Can you work these out from the model? Positions are in its coordinate system, mm. Face numbers are marked on the shaded views. Give positions to 0.01 mm unless a question says otherwise; leave off trailing zeros. Order: outer loops, then holes, each group sorted by start corner. A loop starts at its lowest first (then second) coordinate and runs counter-clockwise, first axis right, second up. Notation, with made-up numbers: (-23, 49) - (12, 49) arc R7 ccw to (12, 60) - close; hole circle Ø7 at (78, 1.25). An arc over 180 degrees is marked (long way). Use one line per item in the form item = value. Start each with the question number.
1) We'd pull the mould along X, two halves only. Please class the marked faces 1, 2, 3 and 4: released by +X, released by -X, zero draft, split by the parting line, or undercut.
2) For pin 1 (6.5 mm diameter, centred on x = -71, z = 9.25, fed in from -Y); pin 2 (1.5 mm diameter, centred on x = -41.5, z = -9.5, fed in from +Y); pin 3 (4.5 mm diameter, centred on x = 71, z = -50.75, fed in from +Y), each with a flat end and sliding along its axis, tell me the tip position at first contact or that it passes through.
3) Suppose I cut it at A-A, the plane x = -71. Write out the boundary of the cut face in (y, z).
4) Suppose I cut it at B-B, the plane y = 3. Write out the boundary of the cut face in (x, z), and give its area (3 significant figures).
5) Please list where these lines run through material, in increasing order: probe 1 along Z at (x, y) = (71, 6); probe 2 along Z at (x, y) = (61.5, 8.25); probe 3 along Z at (x, y) = (-42.5, 4.5).
6) Suppose I cut it at D-D, the plane x = 65. Write out the boundary of the cut face in (y, z).
7) Suppose I cut it at C-C, the plane z = -50.75. Write out the boundary of the cut face in (x, y).
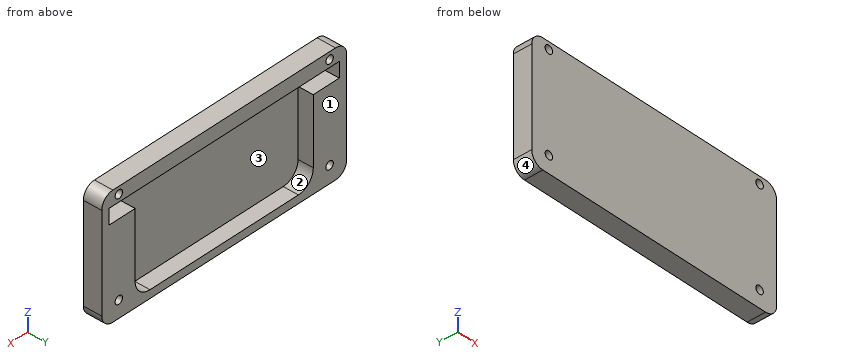
```python
from build123d import *

# Parameters (mm, degrees)
SKETCH_1_W      = 165
SKETCH_1_H      = 75
SKETCH_1_R      = 2.5
EXTRUDE_1_DEPTH = 9.5
EXTRUDE_START   = -2
SKETCH_1_2_W    = 165
SKETCH_1_2_H    = 75
SKETCH_1_2_R    = 2.5
EXTRUDE_2_DEPTH = 2
FILLET_1_R      = 10
FILLET_2_R      = 7.5


with BuildPart() as part:
    # Sketch 1 → Extrude 1 (new body)
    with BuildSketch(Plane(origin=(0, 0, 0), x_dir=(1, 0, 0), z_dir=(0, 1, 0))):
        with Locations((0, 23.75)):
            Rectangle(SKETCH_1_W, SKETCH_1_H)
        with Locations(Location((-71, -9.25, 0), (0, 0, 270))):
            Circle(SKETCH_1_R, mode=Mode.SUBTRACT)
        with Locations(Location((-71, 50.75, 0), (0, 0, 270))):
            Circle(SKETCH_1_R, mode=Mode.SUBTRACT)
        with Locations(Location((71, -9.25, 0), (0, 0, 90))):
            Circle(SKETCH_1_R, mode=Mode.SUBTRACT)
        with Locations(Location((71, 50.75, 0), (0, 0, 90))):
            Circle(SKETCH_1_R, mode=Mode.SUBTRACT)
        Polygon((77.5, -4.75), (-77.5, -4.75), (-77.5, 4.75), (-60, 4.75), (-60, 56.25), (60, 56.25), (60, 4.75), (77.5, 4.75), align=None, mode=Mode.SUBTRACT)
    extrude(amount=EXTRUDE_1_DEPTH)

    # Sketch 1_2 → Extrude 2 (add)
    # profile 1 of 2: a face of its own
    with BuildSketch(Plane(origin=(0, 0, 0), x_dir=(1, 0, 0), z_dir=(0, 1, 0)).offset(EXTRUDE_START)):
        with Locations((0, 23.75)):
            Rectangle(SKETCH_1_2_W, SKETCH_1_2_H)
        with Locations(Location((71, -9.25, 0), (0, 0, 90))):
            Circle(SKETCH_1_2_R, mode=Mode.SUBTRACT)
        with Locations(Location((-71, 50.75, 0), (0, 0, 270))):
            Circle(SKETCH_1_2_R, mode=Mode.SUBTRACT)
        with Locations(Location((-71, -9.25, 0), (0, 0, 270))):
            Circle(SKETCH_1_2_R, mode=Mode.SUBTRACT)
        with Locations(Location((71, 50.75, 0), (0, 0, 90))):
            Circle(SKETCH_1_2_R, mode=Mode.SUBTRACT)
        Polygon((77.5, -4.75), (77.5, 4.75), (60, 4.75), (60, 56.25), (-60, 56.25), (-60, 4.75), (-77.5, 4.75), (-77.5, -4.75), align=None, mode=Mode.SUBTRACT)
    # profile 2 of 2: a face of its own
    with BuildSketch(Plane(origin=(0, 0, 0), x_dir=(1, 0, 0), z_dir=(0, 1, 0)).offset(EXTRUDE_START)):
        Polygon((77.5, -4.75), (-77.5, -4.75), (-77.5, 4.75), (-60, 4.75), (-60, 56.25), (60, 56.25), (60, 4.75), (77.5, 4.75), align=None)
    extrude(amount=EXTRUDE_2_DEPTH)

    # Fillet 1
    fillet_1_edges = [part.edges().sort_by_distance(p)[0] for p in [
        (60, 4.75, -56.25),
        (-60, 4.75, -56.25),
    ]]
    fillet(fillet_1_edges, radius=FILLET_1_R)

    # Fillet 2
    fillet_2_edges = [part.edges().sort_by_distance(p)[0] for p in [
        (-82.5, 3.75, -61.25),
        (82.5, 3.75, -61.25),
        (82.5, 3.75, 13.75),
        (-82.5, 3.75, 13.75),
    ]]
    fillet(fillet_2_edges, radius=FILLET_2_R)


solid = part.part
```
Result sheet:
q1.face_1 = zero draft
q1.face_2 = undercut
q1.face_3 = undercut
q1.face_4 = released by -X
q2.pin_1 = -2
q2.pin_2 = 0
q2.pin_3 = through
q3.outline = (-2, -61.25) - (9.5, -61.25) - (9.5, -53.25) - (-2, -53.25) - close; (-2, -48.25) - (9.5, -48.25) - (9.5, -4.75) - (0, -4.75) - (0, 4.75) - (9.5, 4.75) - (9.5, 6.75) - (-2, 6.75) - close; (-2, 11.75) - (9.5, 11.75) - (9.5, 13.75) - (-2, 13.75) - close
q4.outline = (-82.5, -53.75) arc R7.5 ccw to (-75, -61.25) - (75, -61.25) arc R7.5 ccw to (82.5, -53.75) - (82.5, 6.25) arc R7.5 ccw to (75, 13.75) - (-75, 13.75) arc R7.5 ccw to (-82.5, 6.25) - close; hole (-77.5, -4.75) - (-60, -4.75) - (-60, -46.25) arc R10 ccw to (-50, -56.25) - (50, -56.25) arc R10 ccw to (60, -46.25) - (60, -4.75) - (77.5, -4.75) - (77.5, 4.75) - (-77.5, 4.75) - close; hole circle Ø5 at (-71, -50.75); hole circle Ø5 at (-71, 9.25); hole circle Ø5 at (71, -50.75); hole circle Ø5 at (71, 9.25)
q4.area = 4,640 mm²
q5.probe_1 = -61.25 to -53.25, -48.25 to -4.75, 4.75 to 6.75, 11.75 to 13.75
q5.probe_2 = -61.25 to -4.75, 4.75 to 13.75
q5.probe_3 = -61.25 to -56.25, 4.75 to 13.75
q6.outline = (-2, -61.25) - (9.5, -61.25) - (9.5, -4.75) - (0, -4.75) - (0, 4.75) - (9.5, 4.75) - (9.5, 13.75) - (-2, 13.75) - close
q7.outline = (-82.5, -2) - (-73.5, -2) - (-73.5, 9.5) - (-82.5, 9.5) - close; (-68.5, -2) - (68.5, -2) - (68.5, 9.5) - (58.93, 9.5) - (58.93, 0) - (-58.93, 0) - (-58.93, 9.5) - (-68.5, 9.5) - close; (73.5, -2) - (82.5, -2) - (82.5, 9.5) - (73.5, 9.5) - close
